Job drawing, mm, ordinate dimensions from the low corner. One solid piece. A direction names the side the tool comes from. Give positions to 0.01 mm unless a question says otherwise; leave off trailing zeros. Order: outer loops, then holes, each group sorted by start corner. A loop starts at its lowest first (then second) coordinate and runs counter-clockwise, first axis right, second up. Notation, with made-up numbers: M 15,-4.5 L 21,-4.5 A9 cw 21,12.5 Z; hole C 19.25,-24.5 d9. An arc over 180 degrees is marked long. Use CSV: the item, a comma, the result in double quotes. Start each with the question number.
Item 1: Band-saw the part on C-C on y = 9. Write the cut outline in (x, z).
Item 2: Band-saw the part on A-A on y = 11.75. Write the cut outline in (x, z).
Item 3: Pin check, flat tips, straight feed: P1, Ø0.7, axis at y = 12, z = 2.5, coming from the -X side; P2, Ø1, axis at x = 3.5, y = 1.5, coming from the -Z side. Stop position of each tip, or through.
Item 4: Which spindle directions (+Z, -Z, +X, -X, +Y, -Y) get a long thin tool onto all of the face, cutting with end or side? Do the marked faces 4, 5 and 6. Say none if no direction does.
Item 5: Wall check: line 1 along Y through (x, z) = (2, 1.25); line 2 along Y through (x, z) = (3.55, 2.5); line 3 along X through (y, z) = (12.5, 3.1). Give the ranges that are in metal, low to high.
Item 6: Two-plate mould, pull along Z, no slides. Class the marked faces 1, 2 and 3: pulls with the +Z half, pulls with the -Z half, needs draft (parallel to the pull), parting line crosses it, or undercut.
Item 7: Band-saw the part on B-B on z = 2.75. Write the cut outline in (x, y).
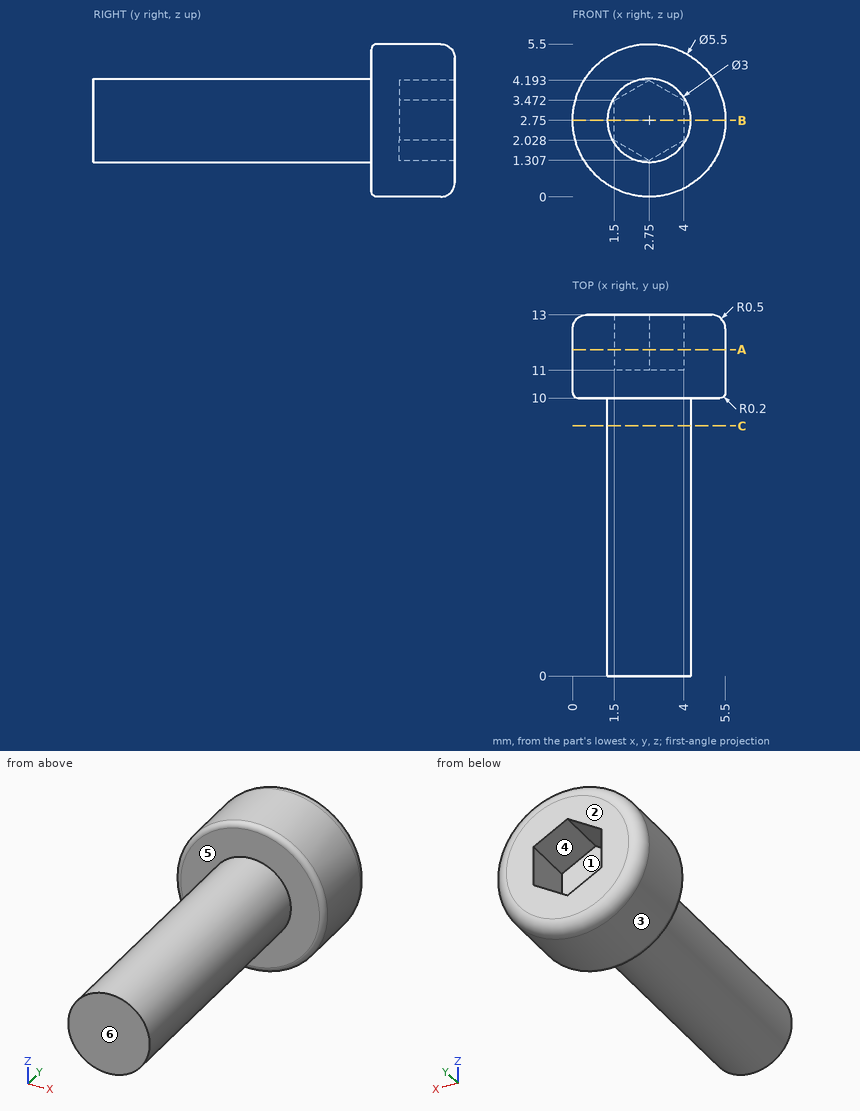
Model answer:
1,outline,"C 2.75,2.75 d3"
2,outline,"C 2.75,2.75 d5.5; hole M 1.5,2.03 L 2.75,1.31 L 4,2.03 L 4,3.47 L 2.75,4.19 L 1.5,3.47 Z"
3,P1,"stops at x = 0"
3,P2,"stops at z = 1.27"
4,face 4,"+Y"
4,face 5,"-Y"
4,face 6,"+Z, -Z, +X, -X, -Y"
5,line 1,"y = 10 to 13"
5,line 2,"y = 0 to 11"
5,line 3,"x = 0.02 to 1.5, 4 to 5.48"
6,face 1,"undercut"
6,face 2,"needs draft"
6,face 3,"parting line crosses it"
7,outline,"M 0,10.2 A0.2 ccw 0.2,10 L 1.25,10 L 1.25,0 L 4.25,0 L 4.25,10 L 5.3,10 A0.2 ccw 5.5,10.2 L 5.5,12.5 A0.5 ccw 5,13 L 4,13 L 4,11 L 1.5,11 L 1.5,13 L 0.5,13 A0.5 ccw 0,12.5 Z"
